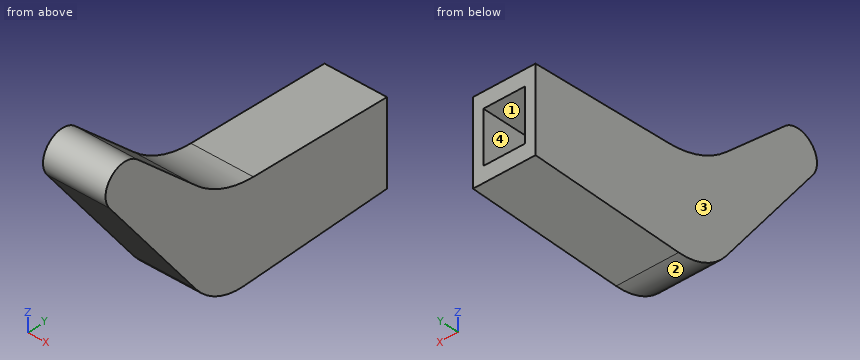
```python
from build123d import *

# Parameters (mm, degrees)
BOSS_EXTRUDE1_DEPTH = 4
BOSS_EXTRUDE2_START = 6
BOSS_EXTRUDE2_DEPTH = 2
BOSS_EXTRUDE3_START = -4
BOSS_EXTRUDE3_DEPTH = 2


with BuildPart() as part:
    # Sketch1 → Boss-Extrude1 (new, symmetric)
    with BuildSketch(Plane(origin=(0, 0, 0), x_dir=(0, 0, -1), z_dir=(1, 0, 0))):
        with BuildLine():
            Line((-5, 0), (-5, 20))
            Line((-5, 20), (-8, 20))
            Line((-8, 20), (-9, -8))
            ThreePointArc((-9, -8), (-10.368373469, -14.408848081), (-13.847540332, -19.962331457))
            Line((-13.847540332, -19.962331457), (-25.002870304, -32.319666758))
            ThreePointArc((-25.002870304, -32.319666758), (-24.977373246, -37.708310367), (-19.609501747, -38.181687186))
            Line((-19.609501747, -38.181687186), (4.253152151, -20))
            ThreePointArc((4.253152151, -20), (7.840921615, -15.576431351), (9, -10))
            Line((9, -10), (8, 20))
            Line((8, 20), (5, 20))
            Line((5, 20), (5, 0))
            ThreePointArc((5, 0), (0, -5), (-5, 0))
        make_face()
    extrude(amount=BOSS_EXTRUDE1_DEPTH, both=True)

    # Sketch1<3> → Boss-Extrude2 (add)
    with BuildSketch(Plane(origin=(0, 0, 0), x_dir=(0, 0, -1), z_dir=(1, 0, 0)).offset(BOSS_EXTRUDE2_START)):
        with BuildLine():
            Line((5, 20), (-5, 20))
            Line((-5, 20), (-5, 0))
            ThreePointArc((-5, 0), (0, 5), (5, 0))
            Line((5, 0), (5, 20))
        make_face()
        with BuildLine():
            Line((-5, 0), (-5, 20))
            Line((-5, 20), (-8, 20))
            Line((-8, 20), (-9, -8))
            ThreePointArc((-9, -8), (-10.368373469, -14.408848081), (-13.847540332, -19.962331457))
            Line((-13.847540332, -19.962331457), (-25.002870304, -32.319666758))
            ThreePointArc((-25.002870304, -32.319666758), (-24.977373246, -37.708310367), (-19.609501747, -38.181687186))
            Line((-19.609501747, -38.181687186), (4.253152151, -20))
            ThreePointArc((4.253152151, -20), (7.840921615, -15.576431351), (9, -10))
            Line((9, -10), (8, 20))
            Line((8, 20), (5, 20))
            Line((5, 20), (5, 0))
            ThreePointArc((5, 0), (0, -5), (-5, 0))
        make_face()
        with BuildLine():
            ThreePointArc((5, 0), (0, 5), (-5, 0))
            Line((-5, 0), (5, 0))
        make_face()
        with BuildLine():
            Line((5, 0), (-5, 0))
            ThreePointArc((-5, 0), (0, -5), (5, 0))
        make_face()
    extrude(amount=-BOSS_EXTRUDE2_DEPTH)

    # Sketch1<4> → Boss-Extrude3 (add)
    with BuildSketch(Plane(origin=(0, 0, 0), x_dir=(0, 0, -1), z_dir=(1, 0, 0)).offset(BOSS_EXTRUDE3_START)):
        with BuildLine():
            ThreePointArc((5, 0), (0, 5), (-5, 0))
            Line((-5, 0), (5, 0))
        make_face()
        with BuildLine():
            Line((5, 0), (-5, 0))
            ThreePointArc((-5, 0), (0, -5), (5, 0))
        make_face()
        with BuildLine():
            Line((5, 20), (-5, 20))
            Line((-5, 20), (-5, 0))
            ThreePointArc((-5, 0), (0, 5), (5, 0))
            Line((5, 0), (5, 20))
        make_face()
        with BuildLine():
            Line((-5, 0), (-5, 20))
            Line((-5, 20), (-8, 20))
            Line((-8, 20), (-9, -8))
            ThreePointArc((-9, -8), (-10.368373469, -14.408848081), (-13.847540332, -19.962331457))
            Line((-13.847540332, -19.962331457), (-25.002870304, -32.319666758))
            ThreePointArc((-25.002870304, -32.319666758), (-24.977373246, -37.708310367), (-19.609501747, -38.181687186))
            Line((-19.609501747, -38.181687186), (4.253152151, -20))
            ThreePointArc((4.253152151, -20), (7.840921615, -15.576431351), (9, -10))
            Line((9, -10), (8, 20))
            Line((8, 20), (5, 20))
            Line((5, 20), (5, 0))
            ThreePointArc((5, 0), (0, -5), (-5, 0))
        make_face()
    extrude(amount=-BOSS_EXTRUDE3_DEPTH)


solid = part.part
```
Input: part model. Units: mm. Frame: model coordinates. Face numbers are marked on the shaded views. Coordinates: 2 decimals unless noted, no trailing zeros. Loops run counter-clockwise (first coordinate to the right, second up) from the corner with the lowest first, then second, coordinate; pieces in that order, holes last. Notation, with made-up numbers: M -8.5,-4 L 48.5,-4 A20 ccw 48.5,33 Z; hole C 75.25,-4.5 d10. An arc over 180 degrees is marked long. Use a Markdown table: item, result. Add a question column.
1) Section A-A, the plane x = 1. Return the cut outline in (y, z), plus the area to 3 significant figures.
2) Line query: L1, parallel to Z at x = -3.75, y = -0.5; L2, parallel to Z at x = 0, y = 2.5 (3 decimals); L3, parallel to Y at x = -1.5, z = 22. Output: solid intervals per line, ascending. Write a range as from..to.
3) Pin query (flat end, axial travel): P1, Ø1.5, axis at x = 1.5, y = 3, coming from the +Z side; P2, Ø2, axis at x = 3.5, y = -1.5, coming from the -Z side; P3, Ø6, axis at x = -0.5, z = 2.5, coming from the -Y side; P4, Ø12, axis at y = -23.5, z = -0.5, coming from the +X side. Return the tip coordinate at first contact, or that it passes through.
4) Section D-D, the plane y = 1.5. Return the cut outline in (x, z), plus the area to 3 significant figures.
5) Section C-C, the plane z = -1. Return the cut outline in (x, y), plus the area to 3 significant figures.
6) Draft query along Z for the marked faces 1, 2, 3 and 4. Return one class per face: +Z half, -Z half, draft (parallel to the pull), parting line (faces both ways), or undercut.
7) Section B-B, the plane y = 8.5. Return the cut outline in (x, z).
Answer below:
| question | item | result |
|---|---|---|
| 1 | outline | M -38.18,19.61 L -20,-4.25 A12.07 ccw -10,-9 L 20,-8 L 20,-5 L 0,-5 A5 cw 0,5 L 20,5 L 20,8 L -8,9 A18.86 cw -19.96,13.85 L -32.32,25 A4 ccw Z |
| 1 | area | 710 mm2 |
| 2 | L1 | -8.68..-4.97, 4.97..8.73 |
| 2 | L2 | -8.583..-5, 5..8.625 |
| 2 | L3 | -39..-28.99 |
| 3 | P1 | z = 8.63 |
| 3 | P2 | z = -8.75 |
| 3 | P3 | y = -27.43 |
| 3 | P4 | x = 6 |
| 4 | outline | M -6,-8.62 L 6,-8.62 L 6,8.66 L -6,8.66 Z; hole M -4,-5 L 4,-5 L 4,5 L -4,5 Z |
| 4 | area | 127 mm2 |
| 5 | outline | M -6,-22.48 L 6,-22.48 L 6,20 L 4,20 L 4,-4.9 L -4,-4.9 L -4,20 L -6,20 Z |
| 5 | area | 311 mm2 |
| 6 | face 1 | undercut |
| 6 | face 2 | -Z half |
| 6 | face 3 | draft |
| 6 | face 4 | undercut |
| 7 | outline | M -6,-8.38 L 6,-8.38 L 6,8.41 L -6,8.41 Z; hole M -4,-5 L 4,-5 L 4,5 L -4,5 Z |
